Here's how the part is built. I have some questions about the finished solid (model axes, mm). Face numbers are marked on the shaded views. A direction names the side the tool comes from. Round coordinates to 2 decimals unless told otherwise and drop trailing zeros. Write each loop counter-clockwise with the first axis right and the second up, starting at its lowest first coordinate (ties: lowest second). Pieces come first, ordered by that corner, then holes. Notation, with made-up numbers: (29.5, 73) -> (70.5, 73) arc R18 cw to (70.5, 97) -> close; hole circle Ø8 at (-18, -27.5). An arc over 180 degrees is marked (long way). Answer in a Markdown table with one row per item.
from build123d import *

# Parameters (mm, degrees)
SKETCH1_W           = 76.2
SKETCH1_H           = 203.2
BOSS_EXTRUDE1_DEPTH = 25.4
CUT_EXTRUDE1_DEPTH  = 219.499061783
FILLET1_R           = 9.525
CHAMFER3_SIZE       = 7.62
CHAMFER5_SIZE       = 12.7
CHAMFER5_SIZE2      = 15.24
SKETCH5_R           = 4.064
CUT_EXTRUDE2_DEPTH  = 6.35
CHAMFER6_SIZE       = 5.08
FILLET2_R           = 9.525
CHAMFER7_SIZE       = 7.62


with BuildPart() as part:
    # Sketch1 → Boss-Extrude1 (new body)
    with BuildSketch(Plane.XY):
        with Locations((38.1, 101.6)):
            Rectangle(SKETCH1_W, SKETCH1_H)
    extrude(amount=BOSS_EXTRUDE1_DEPTH)

    # Sketch2 → Cut-Extrude1 (cut, through all)
    with BuildSketch(Plane.XY.offset(25.4)):
        Polygon((0, 0), (55.88, 0), (55.88, 20.32), (63.5, 20.32), (63.5, 185.42), (30.48, 185.42), (7.62, 127), (0, 127), align=None)
        Polygon((0, 142.378540166), (23.799701674, 203.2), (0, 203.2), align=None)
    extrude(amount=-CUT_EXTRUDE1_DEPTH, mode=Mode.SUBTRACT)

    # Fillet1
    fillet1_edges = [part.edges().sort_by_distance(p)[0] for p in [
        (30.48, 185.42, 12.7),
        (63.5, 185.42, 12.7),
    ]]
    fillet(fillet1_edges, radius=FILLET1_R)

    # Chamfer3
    chamfer3_edges = [part.edges().sort_by_distance(p)[0] for p in [
        (76.2, 203.2, 12.7),
    ]]
    chamfer(chamfer3_edges, length=CHAMFER3_SIZE)

    # Chamfer5
    chamfer5_edges = [part.edges().sort_by_distance(p)[0] for p in [
        (23.799701674, 203.2, 12.7),
    ]]
    chamfer5_side = [part.faces().sort_by_distance(p)[0] for p in [
        (11.899850837, 172.789270083, 12.7),
    ]]
    chamfer(chamfer5_edges, length=CHAMFER5_SIZE, length2=CHAMFER5_SIZE2, reference=chamfer5_side[0])

    # Sketch5 → Cut-Extrude2 (cut)
    with BuildSketch(Plane(origin=(76.2, 0, 0), x_dir=(0, 0, -1), z_dir=(1, 0, 0))):
        with Locations((-12.7, 144.78)):
            Circle(SKETCH5_R)
        with Locations((-12.7, 50.8)):
            Circle(SKETCH5_R)
    extrude(amount=-CUT_EXTRUDE2_DEPTH, mode=Mode.SUBTRACT)

    # Chamfer6
    chamfer6_edges = [part.edges().sort_by_distance(p)[0] for p in [
        (76.2, 144.78, 16.764),
        (76.2, 50.8, 16.764),
    ]]
    chamfer(chamfer6_edges, length=CHAMFER6_SIZE)

    # Fillet2
    # the kernel refuses this fillet: 9.525 mm, written as the material it adds along each edge
    with BuildSketch(Plane(origin=(63.5, 20.32, 25.4), x_dir=(-1, 0, 0), z_dir=(0, 0, -1))) as fillet2_piece_1:
        with BuildLine():
            CenterArc((9.525, 9.33255592), FILLET2_R, 180, 78.463040967)
            Line((0, 9.33255592), (-0.1905, 9.33255592))
            Line((-0.1905, 9.33255592), (-0.1905, 0))
            Line((-0.1905, 0), (0, -0.1905))
            ThreePointArc((0, -0.1905), (3.81, -0.1905), (7.5819, -0.186651118))
            Line((7.5819, -0.186651118), (7.62, 0))
        make_face()
    extrude(amount=25.4)

    # Chamfer7
    chamfer7_edges = [part.edges().sort_by_distance(p)[0] for p in [
        (55.88, 0, 12.7),
    ]]
    chamfer(chamfer7_edges, length=CHAMFER7_SIZE)


solid = part.part
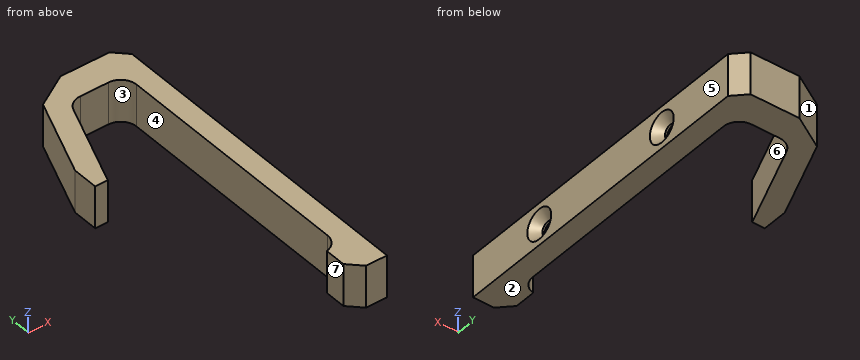
1) We'd pull the mould along Y, two halves only. Please class the marked faces 1, 2 and 3: +Y half, -Y half, draft (parallel to the pull), parting line (faces both ways), or undercut.
Response:
| item | result |
|---|---|
| face 1 | +Y half |
| face 2 | draft |
| face 3 | undercut |
2) Which directions (+Z, -Z, +X, -X, +Y, -Y) give clear straight access to the entire face, cutting with the end or side of a thin tool? Please do the marked faces 4, 5, 6 and 7.
Response:
| item | result |
|---|---|
| face 4 | +Z, -Z |
| face 5 | +Z, -Z, +X, +Y, -Y |
| face 6 | +Z, -Z, -Y |
| face 7 | +Z, -Z, -X, -Y |
3) I want a section at C-C, the plane z = 12.7. List the corners of the cut face in (x, y) for me (3 decimals).
Response:
| item | result |
|---|---|
| outline | (0, 127) -> (7.62, 127) -> (28.111, 179.366) arc R9.525 cw to (36.981, 185.42) -> (53.975, 185.42) arc R9.525 cw to (63.5, 175.895) -> (63.5, 29.653) arc R9.525 cw to (55.88, 20.32) -> (55.88, 7.62) -> (63.5, 0) -> (76.2, 0) -> (76.2, 41.656) -> (71.12, 46.736) -> (69.85, 46.736) -> (69.85, 54.864) -> (71.12, 54.864) -> (76.2, 59.944) -> (76.2, 135.636) -> (71.12, 140.716) -> (69.85, 140.716) -> (69.85, 148.844) -> (71.12, 148.844) -> (76.2, 153.924) -> (76.2, 195.58) -> (68.58, 203.2) -> (39.04, 203.2) -> (19.172, 191.373) -> (0, 142.379) -> close |
4) For pin 1 (4 mm diameter, centred on x = 64, y = 163, fed in from -Z); pin 2 (9.5 mm diameter, centred on y = 50.8, z = 12.7, fed in from -X); pin 3 (4 mm diameter, centred on y = 15, z = 7.5, fed in from -X); pin 4 (1.5 mm diameter, centred on y = 170, z = 16, fed in from -X), each with a flat end and sliding along its axis, tell me the tip position at first contact or that it passes through.
Response:
| item | result |
|---|---|
| pin 1 | stops at z = 0 |
| pin 2 | stops at x = 63.5 |
| pin 3 | stops at x = 55.88 |
| pin 4 | stops at x = 10.51 |
5) I want a section at D-D, the plane x = 15. List the corners of the cut face in (y, z) for me.
Response:
| item | result |
|---|---|
| outline | (145.86, 0) -> (180.71, 0) -> (180.71, 25.4) -> (145.86, 25.4) -> close |
6) I need wall thicknesses on line 1 (Y direction, x = 70.5, z = 12.7); line 2 (Y direction, x = 70.85, z = 12.7); line 3 (X direction, y = 126.5, z = 9.5). Which ranges of each line are inside material? Lowest first, please. Write a range as [from, to].
Response:
| item | result |
|---|---|
| line 1 | y = [0, 46.74], [54.86, 140.72], [148.84, 201.28] |
| line 2 | y = [0, 46.74], [54.86, 140.72], [148.84, 200.93] |
| line 3 | x = [63.5, 76.2] |
7) I want a section at A-A, the plane y = 50.8. List the corners of the cut face in (x, z) for me, and give its area (3 significant figures).
Response:
| item | result |
|---|---|
| outline | (63.5, 0) -> (76.2, 0) -> (76.2, 3.56) -> (71.12, 8.64) -> (69.85, 8.64) -> (69.85, 16.76) -> (71.12, 16.76) -> (76.2, 21.84) -> (76.2, 25.4) -> (63.5, 25.4) -> close |
| area | 245 mm^2 |
8) I want a section at B-B, the plane y = 156. List the corners of the cut face in (x, z) for me.
Response:
| item | result |
|---|---|
| outline | (5.33, 0) -> (18.97, 0) -> (18.97, 25.4) -> (5.33, 25.4) -> close; (63.5, 0) -> (76.2, 0) -> (76.2, 25.4) -> (63.5, 25.4) -> close |
